Read the model definition and answer for the solid it produces. Units are mm, in the model's axes. Face numbers are marked on the shaded views. A direction names the side the tool comes from. Coordinates: 2 decimals unless noted, no trailing zeros. Loops run counter-clockwise (first coordinate to the right, second up) from the corner with the lowest first, then second, coordinate; pieces in that order, holes last. Notation, with made-up numbers: M 74,10.5 L 96,10.5 A15 ccw 96,26.5 Z; hole C -38.75,-9 d3. An arc over 180 degrees is marked long. Use one line per item in the form item = value. Start each with the question number.
1. A tool of negligible diameter and unlimited length cuts with its end or side. For the marked faces 1 and 2, from which of +Z, -Z, +X, -X, +Y, -Y can it reach the whole face along a straight path? Write none if from no direction.
2. Flat-ended cylindrical pins translate along their axes: pin 1 (2 mm diameter, centred on x = -0.5, y = 6, fed in from -Z); pin 2 (1.5 mm diameter, centred on y = 11.5, z = 2, fed in from +X). Find the tip coordinate at first contact, or state that the pin passes through.
3. The part is cut by section A-A (y = 4.25). Give the vertices of the cut face in (x, z), plus the area to 3 significant figures.
4. Find the intervals of material crossed by probe 1 along Y at (x, z) = (-2.25, -0.5); probe 2 along Y at (x, z) = (-0.75, 1.25); probe 3 along X at (y, z) = (2.25, -0.5), in increasing order. Write a range as [from, to].
from build123d import *

# Parameters (mm, degrees)
F0_R     = 1.5
F1_DEPTH = 16
F0_R_2   = 3
F2_DEPTH = 2
F4_SIZE  = 0.5


# Not quite as in the source:
# - a fillet or chamfer that OpenCascade refuses, or shapes differently, is made with other operations: its cross-section is extruded or revolved along the edge and cut away or added


with BuildPart() as f1:
    # F0 (on Front) → F1 (new body)
    with BuildSketch(Plane.XZ):
        Circle(F0_R)
    extrude(amount=-F1_DEPTH)

    # F0 (on Front) → F2 (join)
    with BuildSketch(Plane.XZ):
        Circle(F0_R_2)
        Circle(F0_R, mode=Mode.SUBTRACT)
        Circle(F0_R)
    extrude(amount=F2_DEPTH)

    # F3: fillet of radius 2.5 on 1 edges, made by hand

    # F3_s1 → F3_t2 (revolve, cut)
    with BuildSketch(Plane.XY):
        with BuildLine():
            ThreePointArc((3, 0), (2.1316490873, -1.4364916731), (0.5505102572, -2))
            Line((0.5505102572, -2), (3, -2))
            Line((3, -2), (3, 0))
        make_face()
    revolve(axis=Axis((0, -2, 0), (0, -1, 0)), mode=Mode.SUBTRACT)

    # F4
    f4_edges = [f1.edges().sort_by_distance(p)[0] for p in [
        (-1.5, 16, 0),
    ]]
    chamfer(f4_edges, length=F4_SIZE)


solid = f1.part
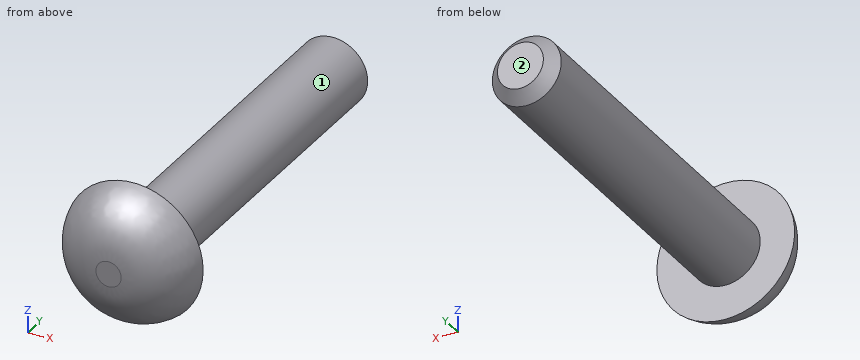
Computed values:
q1.face_1 = +Y
q1.face_2 = +Z, -Z, +X, -X, +Y
q2.pin_1 = -1.5
q2.pin_2 = 0.83
q3.outline = C 0,0 d3
q3.area = 7.07 mm²
q4.probe_1 = [-1.28, 0]
q4.probe_2 = [-1.83, 15.54]
q4.probe_3 = [-1.41, 1.41]
